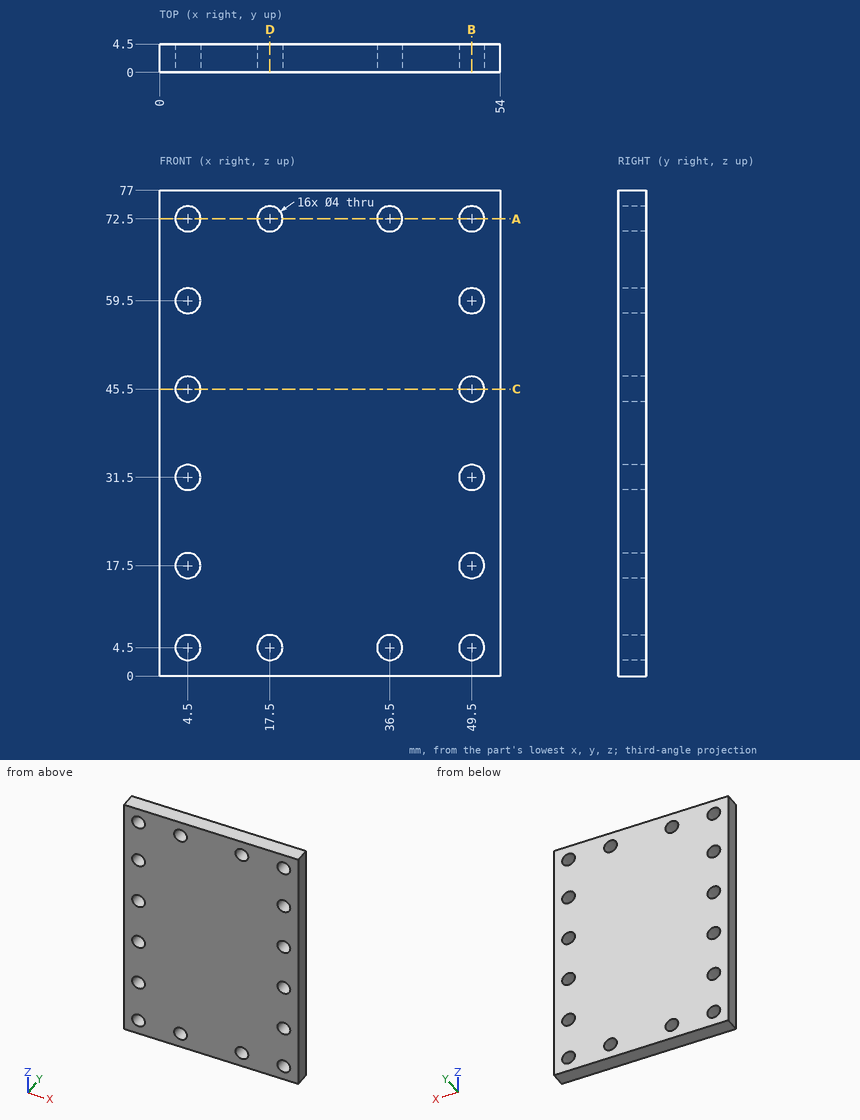
Geometry: see drawing. Coordinates: mm, zero at the bounding-box minimum. Give positions to 0.01 mm unless a question says otherwise; leave off trailing zeros. Write each loop counter-clockwise with the first axis right and the second up, starting at its lowest first coordinate (ties: lowest second). Pieces come first, ordered by that corner, then holes. Notation, with made-up numbers: M -18,23.5 L 27,23.5 A33 cw 27,61.5 Z; hole C 59.5,15.5 d10. An arc over 180 degrees is marked long. Answer in a Markdown table with one row per item. Add a question column.
(1) Section B-B on x = 49.5. Return loops of the section in (y, z), and give its area (4 significant figures).
(2) Section C-C on z = 45.5. Return loops of the section in (x, y).
(3) First-contact query: pin 1 (5 mm diameter, centred on x = 49.5, z = 59.5, fed in from -Y). Flat tip, straight axial feed; report the tip coordinate or a pass-through.
(4) Section A-A on z = 72.5. Return loops of the section in (x, y), and give its area (3 significant figures).
(5) Section D-D on x = 17.5. Return loops of the section in (y, z).
(6) Ray query, line 1 (X direction, y = 3.5, z = 31.5); line 2 (Z direction, x = 17.5, y = 2.7); line 3 (X direction, y = 3.15, z = 72.5). Return the intervals inside material, ascending.
Result set:
| question | item | result |
|---|---|---|
| 1 | outline | M 0,0 L 4.5,0 L 4.5,2.5 L 0,2.5 Z; M 0,6.5 L 4.5,6.5 L 4.5,15.5 L 0,15.5 Z; M 0,19.5 L 4.5,19.5 L 4.5,29.5 L 0,29.5 Z; M 0,33.5 L 4.5,33.5 L 4.5,43.5 L 0,43.5 Z; M 0,47.5 L 4.5,47.5 L 4.5,57.5 L 0,57.5 Z; M 0,61.5 L 4.5,61.5 L 4.5,70.5 L 0,70.5 Z; M 0,74.5 L 4.5,74.5 L 4.5,77 L 0,77 Z |
| 1 | area | 238.5 mm^2 |
| 2 | outline | M 0,0 L 2.5,0 L 2.5,4.5 L 0,4.5 Z; M 6.5,0 L 47.5,0 L 47.5,4.5 L 6.5,4.5 Z; M 51.5,0 L 54,0 L 54,4.5 L 51.5,4.5 Z |
| 3 | pin 1 | stops at y = 0 |
| 4 | outline | M 0,0 L 2.5,0 L 2.5,4.5 L 0,4.5 Z; M 6.5,0 L 15.5,0 L 15.5,4.5 L 6.5,4.5 Z; M 19.5,0 L 34.5,0 L 34.5,4.5 L 19.5,4.5 Z; M 38.5,0 L 47.5,0 L 47.5,4.5 L 38.5,4.5 Z; M 51.5,0 L 54,0 L 54,4.5 L 51.5,4.5 Z |
| 4 | area | 171 mm^2 |
| 5 | outline | M 0,0 L 4.5,0 L 4.5,2.5 L 0,2.5 Z; M 0,6.5 L 4.5,6.5 L 4.5,70.5 L 0,70.5 Z; M 0,74.5 L 4.5,74.5 L 4.5,77 L 0,77 Z |
| 6 | line 1 | x = 0 to 2.5, 6.5 to 47.5, 51.5 to 54 |
| 6 | line 2 | z = 0 to 2.5, 6.5 to 70.5, 74.5 to 77 |
| 6 | line 3 | x = 0 to 2.5, 6.5 to 15.5, 19.5 to 34.5, 38.5 to 47.5, 51.5 to 54 |
